```python
from build123d import *

# Parameters (mm, degrees)
SKETCH1_R           = 5
BOSS_EXTRUDE1_DEPTH = 1.6
SKETCH2_R           = 1.1
CUT_EXTRUDE1_DEPTH  = 80.073130708
CUT_EXTRUDE2_REACH  = 81.073
SKETCH3_R           = 1.6
CUT_EXTRUDE3_REACH  = 81.073
SKETCH5_R           = 1.1


with BuildPart() as part:
    # Sketch1 → Boss-Extrude1 (new body)
    with BuildSketch(Plane(origin=(0, 0, 0), x_dir=(1, 0, 0), z_dir=(0, 1, 0))):
        Polygon((-20, 65), (20, 65), (45, 25), (45, 5), (35, 5), (35, -35), (45, -35), (45, -50), (20, -60), (-20, -60), (-45, -50), (-45, -35), (-35, -35), (-35, 5), (-45, 5), (-45, 25), align=None)
        with Locations(Location((0, 42.914947937, 0), (0, 0, 270))):
            Circle(SKETCH1_R, mode=Mode.SUBTRACT)
    extrude(amount=BOSS_EXTRUDE1_DEPTH)

    # Sketch2 → Cut-Extrude1 (cut, through all)
    with BuildSketch(Plane(origin=(0, 1.6, 0), x_dir=(1, 0, 0), z_dir=(0, 1, 0))):
        with Locations(Location((-20, -6, 0), (0, 0, 270))):
            Circle(SKETCH2_R)
        with Locations(Location((-20, -24, 0), (0, 0, 90))):
            Circle(SKETCH2_R)
        with Locations(Location((20, -24, 0), (0, 0, 270))):
            Circle(SKETCH2_R)
        with Locations(Location((20, -6, 0), (0, 0, 90))):
            Circle(SKETCH2_R)
    extrude(amount=-CUT_EXTRUDE1_DEPTH, mode=Mode.SUBTRACT)

    # Sketch3 → Cut-Extrude2 (cut, up to next)
    with BuildSketch(Plane(origin=(0, 1.6, 0), x_dir=(1, 0, 0), z_dir=(0, 1, 0)), mode=Mode.PRIVATE) as cut_extrude2_sk1:
        with Locations(Location((-20, 26.581871199, 0), (0, 0, 270))):
            Circle(SKETCH3_R)
    cut_extrude2_tool1 = extrude(cut_extrude2_sk1.sketch, amount=-CUT_EXTRUDE2_REACH, mode=Mode.PRIVATE) & part.part
    # Sketch3 → Cut-Extrude2 (cut, up to next)
    with BuildSketch(Plane(origin=(0, 1.6, 0), x_dir=(1, 0, 0), z_dir=(0, 1, 0)), mode=Mode.PRIVATE) as cut_extrude2_sk2:
        with Locations(Location((20, 26.581871199, 0), (0, 0, 270))):
            Circle(SKETCH3_R)
    cut_extrude2_tool2 = extrude(cut_extrude2_sk2.sketch, amount=-CUT_EXTRUDE2_REACH, mode=Mode.PRIVATE) & part.part
    # Sketch3 → Cut-Extrude2 (cut, up to next)
    with BuildSketch(Plane(origin=(0, 1.6, 0), x_dir=(1, 0, 0), z_dir=(0, 1, 0)), mode=Mode.PRIVATE) as cut_extrude2_sk3:
        with Locations(Location((20, 6.581871199, 0), (0, 0, 270))):
            Circle(SKETCH3_R)
    cut_extrude2_tool3 = extrude(cut_extrude2_sk3.sketch, amount=-CUT_EXTRUDE2_REACH, mode=Mode.PRIVATE) & part.part
    # Sketch3 → Cut-Extrude2 (cut, up to next)
    with BuildSketch(Plane(origin=(0, 1.6, 0), x_dir=(1, 0, 0), z_dir=(0, 1, 0)), mode=Mode.PRIVATE) as cut_extrude2_sk4:
        with Locations(Location((-20, 6.581871199, 0), (0, 0, 270))):
            Circle(SKETCH3_R)
    cut_extrude2_tool4 = extrude(cut_extrude2_sk4.sketch, amount=-CUT_EXTRUDE2_REACH, mode=Mode.PRIVATE) & part.part
    add(cut_extrude2_tool1.solids().sort_by_distance((-20, 1.6, -26.581871))[0], mode=Mode.SUBTRACT)
    add(cut_extrude2_tool2.solids().sort_by_distance((20, 1.6, -26.581871))[0], mode=Mode.SUBTRACT)
    add(cut_extrude2_tool3.solids().sort_by_distance((20, 1.6, -6.581871))[0], mode=Mode.SUBTRACT)
    add(cut_extrude2_tool4.solids().sort_by_distance((-20, 1.6, -6.581871))[0], mode=Mode.SUBTRACT)

    # Sketch5 → Cut-Extrude3 (cut, up to next)
    with BuildSketch(Plane(origin=(0, 1.6, 0), x_dir=(1, 0, 0), z_dir=(0, 1, 0)), mode=Mode.PRIVATE) as cut_extrude3_sk1:
        with Locations(Location((-36.412283149, 8, 0), (0, 0, 270))):
            Circle(SKETCH5_R)
    cut_extrude3_tool1 = extrude(cut_extrude3_sk1.sketch, amount=-CUT_EXTRUDE3_REACH, mode=Mode.PRIVATE) & part.part
    # Sketch5 → Cut-Extrude3 (cut, up to next)
    with BuildSketch(Plane(origin=(0, 1.6, 0), x_dir=(1, 0, 0), z_dir=(0, 1, 0)), mode=Mode.PRIVATE) as cut_extrude3_sk2:
        with Locations(Location((36.412283149, 8, 0), (0, 0, 270))):
            Circle(SKETCH5_R)
    cut_extrude3_tool2 = extrude(cut_extrude3_sk2.sketch, amount=-CUT_EXTRUDE3_REACH, mode=Mode.PRIVATE) & part.part
    # Sketch5 → Cut-Extrude3 (cut, up to next)
    with BuildSketch(Plane(origin=(0, 1.6, 0), x_dir=(1, 0, 0), z_dir=(0, 1, 0)), mode=Mode.PRIVATE) as cut_extrude3_sk3:
        with Locations(Location((-14.134917172, 42.301953571, 0), (0, 0, 270))):
            Circle(SKETCH5_R)
    cut_extrude3_tool3 = extrude(cut_extrude3_sk3.sketch, amount=-CUT_EXTRUDE3_REACH, mode=Mode.PRIVATE) & part.part
    # Sketch5 → Cut-Extrude3 (cut, up to next)
    with BuildSketch(Plane(origin=(0, 1.6, 0), x_dir=(1, 0, 0), z_dir=(0, 1, 0)), mode=Mode.PRIVATE) as cut_extrude3_sk4:
        with Locations(Location((14.134917172, 42.301953571, 0), (0, 0, 270))):
            Circle(SKETCH5_R)
    cut_extrude3_tool4 = extrude(cut_extrude3_sk4.sketch, amount=-CUT_EXTRUDE3_REACH, mode=Mode.PRIVATE) & part.part
    add(cut_extrude3_tool1.solids().sort_by_distance((-36.412283, 1.6, -8))[0], mode=Mode.SUBTRACT)
    add(cut_extrude3_tool2.solids().sort_by_distance((36.412283, 1.6, -8))[0], mode=Mode.SUBTRACT)
    add(cut_extrude3_tool3.solids().sort_by_distance((-14.134917, 1.6, -42.301954))[0], mode=Mode.SUBTRACT)
    add(cut_extrude3_tool4.solids().sort_by_distance((14.134917, 1.6, -42.301954))[0], mode=Mode.SUBTRACT)


solid = part.part
```
Read the model definition and answer for the solid it produces. Units are mm, in the model's axes. Round coordinates to 2 decimals unless told otherwise and drop trailing zeros. Write each loop counter-clockwise with the first axis right and the second up, starting at its lowest first coordinate (ties: lowest second). Pieces come first, ordered by that corner, then holes. Notation, with made-up numbers: (21, -11) - (44, -11) arc R24 ccw to (44, 14) - close; hole circle Ø10 at (-33.75, -26.5). An arc over 180 degrees is marked (long way). One line per item, written item: value.
Q1. For a pull along X with two mould halves and no side action, classify faces 1 (the cylindrical face through (-18.414, 0.811, -6.79)), 2 (the cylindrical face through (21.586, 0.811, -6.79)), 3 (the flat face through (1, 0, -3)), 4 (the flat face through (32.67, 0.79, 54.93)) as pulls with the +X half, pulls with the -X half, needs draft (parallel to the pull), parting line crosses it, or undercut.
The answers:
face 1: undercut
face 2: undercut
face 3: needs draft
face 4: pulls with the +X half
Q2. Straight lines are drawn through the part: line 1 (X direction, y = 0.85, z = 24); line 2 (X direction, y = 1.3, z = -8.5); line 3 (Z direction, x = -2.5, y = 1.35). For each, find the intervals that lie inside material, in ascending order. Write a range as from..to.
The answers:
line 1: x = -35..-21.1, -18.9..18.9, 21.1..35
line 2: x = -45..-37.39, -35.43..35.43, 37.39..45
line 3: z = -65..-47.25, -38.58..60
Q3. Find section A-A (x = 0). Determine the outline of the cut face in (y, z).
The answers:
outline: (0, -65) - (1.6, -65) - (1.6, -47.91) - (0, -47.91) - close; (0, -37.91) - (1.6, -37.91) - (1.6, 60) - (0, 60) - close
Q4. Find section C-C (z = -53). Determine the outline of the cut face in (x, y).
The answers:
outline: (-27.5, 0) - (27.5, 0) - (27.5, 1.6) - (-27.5, 1.6) - close
Q5. Each of these flat-tipped pins is pushed along its axis until it touches: P1, Ø1.5, axis at x = 16.5, z = 11, coming from the -Y side; P2, Ø0.5, axis at y = 1, z = 12, coming from the -X side; P3, Ø2, axis at x = 20, z = 6, coming from the +Y side; P4, Ø0.5, axis at x = 40.5, y = 1, coming from the +Z side. Where does it stop, or does it pass through?
The answers:
P1: stops at y = 0
P2: stops at x = -35
P3: passes through
P4: stops at z = 51.9
Q6. Find section D-D (x = 23.5). Determine the outline of the cut face in (y, z), and give its area (3 significant figures).
The answers:
outline: (0, -59.4) - (1.6, -59.4) - (1.6, 58.6) - (0, 58.6) - close
area: 189 mm2
Q7. Find section B-B (y = 0.6). Count the separate pieces of the cut face and the enclosed holes in it, and give its area (3 significant figures).
The answers:
separate pieces: 1
enclosed holes: 13
area: 9,060 mm2
